Geometry check sheet. Reference: the model listing, model coordinates, mm. A direction names the side the tool comes from. Round coordinates to 2 decimals unless told otherwise and drop trailing zeros. Write each loop counter-clockwise with the first axis right and the second up, starting at its lowest first coordinate (ties: lowest second). Pieces come first, ordered by that corner, then holes. Notation, with made-up numbers: M -21.5,-36 L 13.5,-36 A9 ccw 13.5,-30 Z; hole C 45.5,-11.75 d8. An arc over 180 degrees is marked long. One line per item, written item: value. Start each with the question number.
1. Release check for a two-part mould opening along Y. For faces 3 (the flat face through (-8, 0, 286)), 4 (the flat face through (0, -10, 286)), 5 (the flat face through (0, 10, 286)) record: pulls with the +Y half, pulls with the -Y half, needs draft (parallel to the pull), parting line crosses it, or undercut.
2. Depth check by flat-ended pin: P1, Ø2.5, axis at x = 0, z = 426, coming from the -Y side; P2, Ø5.5, axis at x = 0, z = 126, coming from the -Y side. Enter the tip coordinate at first touch or a pass-through.
3. Access from +Z, -Z, +X, -X, +Y, -Y to the whole of each face (thin tool, end or side, straight path). Record for faces 1 (the flat face through (0, -8, 286)), 2 (the flat face through (-9, 0, 580)).
4. Section check A-A (z = 383.5). Record the boundary of the cut face in (x, y).
5. Scan lines: probe 1 along X at (y, z) = (8.7, 454); probe 2 along Y at (x, z) = (-1.5, 367). Record each from-to range of solid material in increasing order. Write a range as [from, to].
from build123d import *

# Parameters (mm, degrees)
SKETCH_1_W          = 20
SKETCH_1_H          = 20
SKETCH_1_W_2        = 16
SKETCH_1_H_2        = 16
EXTRUDE_1_DEPTH     = 580
SKETCH_2_R          = 2.1
CUT_EXTRUDE_1_DEPTH = 20
SKETCH_3_R          = 2.1
CUT_EXTRUDE_2_DEPTH = 581.430874437


with BuildPart() as part:
    # 草图1 → 凸台-拉伸1 (new body)
    with BuildSketch(Plane.XY):
        Rectangle(SKETCH_1_W, SKETCH_1_H)
        Rectangle(SKETCH_1_W_2, SKETCH_1_H_2, mode=Mode.SUBTRACT)
    extrude(amount=EXTRUDE_1_DEPTH)

    # 草图2 → 切除-拉伸1 (cut)
    with BuildSketch(Plane(origin=(0, 10, 0), x_dir=(1, 0, 0), z_dir=(0, 1, 0))):
        with Locations(Location((0, -10, 0), (0, 0, 270))):
            Circle(SKETCH_2_R)
        with Locations(Location((0, -126, 0), (0, 0, 270))):
            Circle(SKETCH_2_R)
        with Locations(Location((0, -154, 0), (0, 0, 270))):
            Circle(SKETCH_2_R)
    cut_extrude_1 = extrude(amount=-CUT_EXTRUDE_1_DEPTH, mode=Mode.SUBTRACT)

    # 镜向1: 切除-拉伸1 across plane
    add(cut_extrude_1.mirror(Plane.XY.offset(290)), mode=Mode.SUBTRACT)

    # 草图3 → 切除-拉伸2 (cut, through all)
    with BuildSketch(Plane(origin=(10, 0, 0), x_dir=(0, 0, -1), z_dir=(1, 0, 0))):
        with Locations((-570, 0)):
            Circle(SKETCH_3_R)
        with Locations((-10, 0)):
            Circle(SKETCH_3_R)
        with Locations((-454, 0)):
            Circle(SKETCH_3_R)
        with Locations((-426, 0)):
            Circle(SKETCH_3_R)
        with Locations(Location((-126, 0, 0), (0, 0, 180))):
            Circle(SKETCH_3_R)
        with Locations(Location((-154, 0, 0), (0, 0, 180))):
            Circle(SKETCH_3_R)
    extrude(amount=-CUT_EXTRUDE_2_DEPTH, mode=Mode.SUBTRACT)


solid = part.part
Result sheet:
1. face 3: undercut
1. face 4: pulls with the -Y half
1. face 5: pulls with the +Y half
2. P1: passes through
2. P2: stops at y = -10
3. face 1: +Z, -Z
3. face 2: +Z, +X, -X, +Y, -Y
4. outline: M -10,-10 L 10,-10 L 10,10 L -10,10 Z; hole M -8,-8 L 8,-8 L 8,8 L -8,8 Z
5. probe 1: x = [-10, -2.1], [2.1, 10]
5. probe 2: y = [-10, -8], [8, 10]
